from build123d import *

# Parameters (mm, degrees)
BOSS_EXTRUDE3_DEPTH = 7.62


with BuildPart() as part:
    # Sketch3 → Boss-Extrude3 (new body)
    with BuildSketch(Plane(origin=(0, 0, 0), x_dir=(1, 0, 0), z_dir=(0, 1, 0))):
        with BuildLine():
            ThreePointArc((-1.5875, 4.490128061), (0, 4.7625), (1.5875, 4.490128061))
            Line((1.5875, 4.490128061), (1.5875, 6.35))
            Line((1.5875, 6.35), (-1.5875, 6.35))
            Line((-1.5875, 6.35), (-1.5875, 4.490128061))
        make_face()
        with BuildLine():
            Line((-6.35, -1.5875), (-4.490128061, -1.5875))
            ThreePointArc((-4.490128061, -1.5875), (-4.7625, 0), (-4.490128061, 1.5875))
            Line((-4.490128061, 1.5875), (-6.35, 1.5875))
            Line((-6.35, 1.5875), (-6.35, -1.5875))
        make_face()
        with BuildLine():
            Line((-4.490128061, 1.5875), (-2.749630657, 1.5875))
            ThreePointArc((-2.749630657, 1.5875), (-2.24506403, 2.24506403), (-1.5875, 2.749630657))
            Line((-1.5875, 2.749630657), (-1.5875, 4.490128061))
            ThreePointArc((-1.5875, 4.490128061), (-3.367596045, 3.367596045), (-4.490128061, 1.5875))
        make_face()
        with BuildLine():
            Line((-4.490128061, -1.5875), (-2.749630657, -1.5875))
            ThreePointArc((-2.749630657, -1.5875), (-3.175, 0), (-2.749630657, 1.5875))
            Line((-2.749630657, 1.5875), (-4.490128061, 1.5875))
            ThreePointArc((-4.490128061, 1.5875), (-4.7625, 0), (-4.490128061, -1.5875))
        make_face()
        with BuildLine():
            ThreePointArc((-1.5875, 2.749630657), (0, 3.175), (1.5875, 2.749630657))
            Line((1.5875, 2.749630657), (1.5875, 4.490128061))
            ThreePointArc((1.5875, 4.490128061), (0, 4.7625), (-1.5875, 4.490128061))
            Line((-1.5875, 4.490128061), (-1.5875, 2.749630657))
        make_face()
        with BuildLine():
            ThreePointArc((1.5875, 2.749630657), (2.24506403, 2.24506403), (2.749630657, 1.5875))
            Line((2.749630657, 1.5875), (4.490128061, 1.5875))
            ThreePointArc((4.490128061, 1.5875), (3.367596045, 3.367596045), (1.5875, 4.490128061))
            Line((1.5875, 4.490128061), (1.5875, 2.749630657))
        make_face()
        with BuildLine():
            ThreePointArc((4.7625, 0), (4.69391314, -0.805348174), (4.490128061, -1.5875))
            Line((4.490128061, -1.5875), (6.35, -1.5875))
            Line((6.35, -1.5875), (6.35, 1.5875))
            Line((6.35, 1.5875), (4.490128061, 1.5875))
            ThreePointArc((4.490128061, 1.5875), (4.69391314, 0.805348174), (4.7625, 0))
        make_face()
        with BuildLine():
            ThreePointArc((3.175, 0), (3.066814498, -0.821750468), (2.749630657, -1.5875))
            Line((2.749630657, -1.5875), (4.490128061, -1.5875))
            ThreePointArc((4.490128061, -1.5875), (4.69391314, -0.805348174), (4.7625, 0))
            ThreePointArc((4.7625, 0), (4.69391314, 0.805348174), (4.490128061, 1.5875))
            Line((4.490128061, 1.5875), (2.749630657, 1.5875))
            ThreePointArc((2.749630657, 1.5875), (3.066814498, 0.821750468), (3.175, 0))
        make_face()
        with BuildLine():
            Line((-1.5875, -4.490128061), (-1.5875, -2.749630657))
            ThreePointArc((-1.5875, -2.749630657), (-1.81637725, -2.604111881), (-2.032, -2.439590334))
            ThreePointArc((-2.032, -2.439590334), (-2.428479446, -2.045265895), (-2.749630657, -1.5875))
            Line((-2.749630657, -1.5875), (-4.490128061, -1.5875))
            ThreePointArc((-4.490128061, -1.5875), (-3.367596045, -3.367596045), (-1.5875, -4.490128061))
        make_face()
        with BuildLine():
            Line((-1.5875, -2.749630657), (-1.5875, -2.439590334))
            Line((-1.5875, -2.439590334), (-2.032, -2.439590334))
            ThreePointArc((-2.032, -2.439590334), (-1.81637725, -2.604111881), (-1.5875, -2.749630657))
        make_face()
        with BuildLine():
            Line((1.5875, -2.749630657), (1.5875, -2.439590334))
            Line((1.5875, -2.439590334), (-1.5875, -2.439590334))
            Line((-1.5875, -2.439590334), (-1.5875, -2.749630657))
            ThreePointArc((-1.5875, -2.749630657), (0, -3.175), (1.5875, -2.749630657))
        make_face()
        with BuildLine():
            ThreePointArc((1.5875, -2.749630657), (1.81637725, -2.604111881), (2.032, -2.439590334))
            Line((2.032, -2.439590334), (1.5875, -2.439590334))
            Line((1.5875, -2.439590334), (1.5875, -2.749630657))
        make_face()
        with BuildLine():
            ThreePointArc((2.749630657, -1.5875), (2.428479446, -2.045265895), (2.032, -2.439590334))
            ThreePointArc((2.032, -2.439590334), (1.81637725, -2.604111881), (1.5875, -2.749630657))
            Line((1.5875, -2.749630657), (1.5875, -4.490128061))
            ThreePointArc((1.5875, -4.490128061), (3.367596045, -3.367596045), (4.490128061, -1.5875))
            Line((4.490128061, -1.5875), (2.749630657, -1.5875))
        make_face()
        with BuildLine():
            Line((1.5875, -4.490128061), (1.5875, -2.749630657))
            ThreePointArc((1.5875, -2.749630657), (0, -3.175), (-1.5875, -2.749630657))
            Line((-1.5875, -2.749630657), (-1.5875, -4.490128061))
            ThreePointArc((-1.5875, -4.490128061), (0, -4.7625), (1.5875, -4.490128061))
        make_face()
        with BuildLine():
            Line((1.5875, -6.35), (1.5875, -4.490128061))
            ThreePointArc((1.5875, -4.490128061), (0, -4.7625), (-1.5875, -4.490128061))
            Line((-1.5875, -4.490128061), (-1.5875, -6.35))
            Line((-1.5875, -6.35), (1.5875, -6.35))
        make_face()
    extrude(amount=BOSS_EXTRUDE3_DEPTH)


solid = part.part
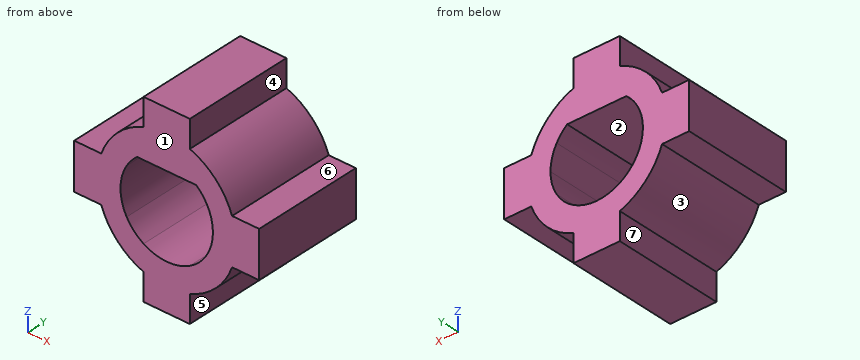
Geometry check sheet. Reference: the model listing, model coordinates, mm. Face numbers are marked on the shaded views. A direction names the side the tool comes from. Round coordinates to 2 decimals unless told otherwise and drop trailing zeros. Loops run counter-clockwise (first coordinate to the right, second up) from the corner with the lowest first, then second, coordinate; pieces in that order, holes last.
Item 1: Access from +Z, -Z, +X, -X, +Y, -Y to the whole of each face (thin tool, end or side, straight path). Record for the marked faces 5, 6 and 7.
Item 2: Cross-section at C-C on z = 5.5. Record the boundary of the cut face in (x, y), then the cut area to 3 significant figures.
Item 3: Cross-section at D-D on x = 0.75. Record the boundary of the cut face in (y, z), then the cut area to 3 significant figures.
Item 4: Gauge pin test, flat ends, axial feed: pin 1 (2 mm diameter, centred on x = -5, y = 5.5, fed in from -Z); pin 2 (1.5 mm diameter, centred on y = 2, z = 5, fed in from -X); pin 3 (3 mm diameter, centred on y = 2, z = 4, fed in from +X). Record the tip position at first contact, or that the pin passes through.
Item 5: Cross-section at B-B on x = 2.25. Record the boundary of the cut face in (y, z), then the cut area to 3 significant figures.
Item 6: Thickness scan on line 1 (Z direction, x = 0, y = 5) (3 decimals); line 2 (X direction, y = 6.5, z = 1); line 3 (Z direction, x = 0.5, y = 4.5). Record the ranges inside material, lowest first.
Item 7: Mould release check, pull along X, two halves, no side actions. Record for the marked faces 1, 2, 3 and 4: pulls with the +X half, pulls with the -X half, needs draft (parallel to the pull), parting line crosses it, or undercut.
Answer sheet:
1. face 5: -Z, +X, +Y, -Y
1. face 6: +Z, +X, +Y, -Y
1. face 7: -Z, -X, +Y, -Y
2. outline: (-1.59, 0) - (1.59, 0) - (1.59, 7.62) - (-1.59, 7.62) - close
2. area: 24.2 mm2
3. outline: (0, -6.35) - (7.62, -6.35) - (7.62, -3.09) - (0, -3.09) - close; (0, 2.44) - (7.62, 2.44) - (7.62, 6.35) - (0, 6.35) - close
3. area: 54.7 mm2
4. pin 1: stops at z = -2.58
4. pin 2: stops at x = -2.15
4. pin 3: stops at x = 4.05
5. outline: (0, -4.2) - (7.62, -4.2) - (7.62, -2.24) - (0, -2.24) - close; (0, 2.24) - (7.62, 2.24) - (7.62, 4.2) - (0, 4.2) - close
5. area: 29.8 mm2
6. line 1: z = -6.35 to -3.175, 2.44 to 6.35
6. line 2: x = -6.35 to -3.01, 3.01 to 6.35
6. line 3: z = -6.35 to -3.14, 2.44 to 6.35
7. face 1: needs draft
7. face 2: undercut
7. face 3: pulls with the -X half
7. face 4: pulls with the +X half
